```python
from build123d import *

# Parameters (mm, degrees)
BOSS_EXTRUDE1_DEPTH = 19
CUT_EXTRUDE1_DEPTH  = 14
CUT_EXTRUDE2_DEPTH  = 4.5
BOSS_EXTRUDE2_DEPTH = 4


with BuildPart() as part:
    # Sketch1 → Boss-Extrude1 (new body, symmetric)
    with BuildSketch(Plane.XY):
        Polygon((0, 0), (0, 36), (5.5, 36), (36, 5.5), (36, 0), align=None)
    extrude(amount=BOSS_EXTRUDE1_DEPTH, both=True)

    # Sketch2 → Cut-Extrude1 (cut, symmetric)
    with BuildSketch(Plane.XY):
        Polygon((5.5, 36), (5.5, 5.5), (36, 5.5), align=None)
    extrude(amount=CUT_EXTRUDE1_DEPTH, both=True, mode=Mode.SUBTRACT)

    # Sketch3 → Cut-Extrude2 (cut, symmetric)
    with BuildSketch(Plane.XY):
        Polygon((0, 29.5), (5.5, 29.5), (5.5, 9), (0, 3.5), align=None)
        Polygon((9, 5.5), (29.5, 5.5), (29.5, 0), (3.5, 0), align=None)
    extrude(amount=CUT_EXTRUDE2_DEPTH, both=True, mode=Mode.SUBTRACT)

    # Sketch4 → Boss-Extrude2 (add, symmetric)
    with BuildSketch(Plane.XY):
        Polygon((0.714757963, -2.5), (-0.201070953, -1.5696698), (1.234750477, 0), (3.535533906, 0), align=None)
        Polygon((0, 3.535533906), (-2.5, 0.714757963), (-1.5696698, -0.201070953), (0, 1.234750477), align=None)
        Polygon((0, 35.3), (0, 32.999216572), (-1.5696698, 31.563395141), (-2.5, 32.479224057), align=None)
        Polygon((32.999216572, 0), (31.563395141, -1.5696698), (32.479224057, -2.5), (35.3, 0), align=None)
    extrude(amount=BOSS_EXTRUDE2_DEPTH, both=True)


solid = part.part
```
For this review, take the finished solid that the model builds, in its own axes (mm). A direction names the side the tool comes from. Round coordinates to 2 decimals unless told otherwise and drop trailing zeros. Write each loop counter-clockwise with the first axis right and the second up, starting at its lowest first coordinate (ties: lowest second). Pieces come first, ordered by that corner, then holes. Notation, with made-up numbers: (47.5, -29.5) - (54.5, -29.5) arc R18 cw to (54.5, -25.5) - close; hole circle Ø11 at (8.25, 30). An arc over 180 degrees is marked (long way). Answer as CSV lines item,"result". Start each with the question number.
(1) Add section A-A, the plane y = 22. State the section outline as (x, z) points, plus the area to 4 significant figures.
(2) Machinability: for faces 1 (the flat face through (5.5, 21, 6)), 2 (the flat face through (3, 29.5, 0)), 3 (the flat face through (17, 3, 4.5)), 4 (the flat face through (-1, 1, -4)), 5 (the flat face through (-1.233, 2.145, -0.056)), which of the approach directions +Z, -Z, +X, -X, +Y, -Y give a long, thin tool a straight path to every point of the face, cutting with its end or side? Answer none if there is none.
(3) Add section C-C, the plane z = 11. State the section outline as (x, y) points.
(4) Mouldability with a two-part tool opening along X and no side actions: class faces 6 (the flat face through (3, 17, -4.5)), 7 (the flat face through (17, 3, -4.5)), 8 (the flat face through (-1.27, 33.87, -0.06)), 9 (the flat face through (29.5, 3, 0)) as +X half, -X half, draft (parallel to the pull), parting line (faces both ways), or undercut.
(5) For line 1 (Z direction, x = 14.5, y = 15.5); line 2 (Y direction, x = 31, z = 0); line 3 (Z direction, x = 20, y = 1), list the stretches that pass through material, from the lowest coordinate up.
(6) Add section B-B, the plane x = 28. State the section outline as (y, z) points, plus the area to 4 significant figures.
(7) For pin 1 (1 mm diameter, centred on x = 31.5, z = -3, fed in from -Y); pin 2 (11 mm diameter, centred on x = 16, z = -2, fed in from -Y); pin 3 (0.8 mm diameter, centred on x = 1.5, y = -1.5, fed in from +Z), all flat-tipped, find the tip position at first contact; note any pin that passes through.
(8) Add section D-D, the plane z = 15. State the section outline as (x, y) points.
From the geometry:
1,outline,"(0, -19) - (19.5, -19) - (19.5, -14) - (5.5, -14) - (5.5, -4.5) - (0, -4.5) - close; (0, 4.5) - (5.5, 4.5) - (5.5, 14) - (19.5, 14) - (19.5, 19) - (0, 19) - close"
1,area,"299.5 mm²"
2,face 1,"+X, +Y"
2,face 2,"+X, -X"
2,face 3,"-Y"
2,face 4,"-Z, -X, +Y, -Y"
2,face 5,"+Z, -Z, -X"
3,outline,"(0, 0) - (36, 0) - (36, 5.5) - (5.5, 5.5) - (5.5, 36) - (0, 36) - close"
4,face 6,"draft"
4,face 7,"undercut"
4,face 8,"-X half"
4,face 9,"undercut"
5,line 1,"z = -19 to -14, 14 to 19"
5,line 2,"y = 0 to 5.5"
5,line 3,"z = -19 to -4.5, 4.5 to 19"
6,outline,"(0, -19) - (13.5, -19) - (13.5, -14) - (5.5, -14) - (5.5, -4.5) - (0, -4.5) - close; (0, 4.5) - (5.5, 4.5) - (5.5, 14) - (13.5, 14) - (13.5, 19) - (0, 19) - close"
6,area,"239.5 mm²"
7,pin 1,"stops at y = -2.01"
7,pin 2,"stops at y = 0"
7,pin 3,"stops at z = 4"
8,outline,"(0, 0) - (36, 0) - (36, 5.5) - (5.5, 36) - (0, 36) - close"
